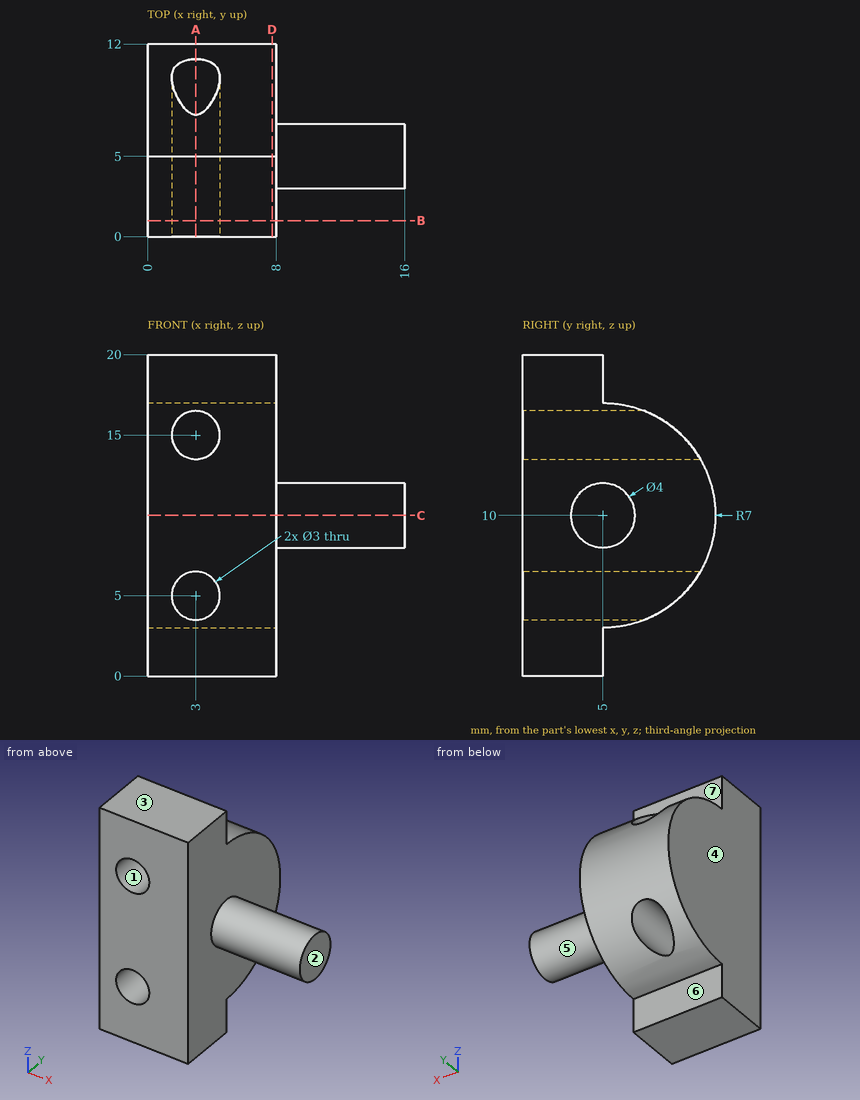
Study the drawing (mm; zero at the part's minimum x, y, z) and answer. A direction names the side the tool comes from. Coordinates: 2 decimals unless noted, no trailing zeros. Loops run counter-clockwise (first coordinate to the right, second up) from the corner with the lowest first, then second, coordinate; pieces in that order, holes last. Notation, with made-up numbers: (-38.75, -40) -> (-20.75, -40) arc R28 cw to (-20.75, -8) -> close; hole circle Ø2 at (1, 11.5). An arc over 180 degrees is marked (long way). Answer as CSV lines item,"result".
1) The part is cut by section D-D (x = 7.75). Give the vertices of the cut face in (y, z).
A:
outline,"(0, 0) -> (5, 0) -> (5, 3) arc R7 ccw to (5, 17) -> (5, 20) -> (0, 20) -> close"
2) For the marked faces 4, 5, 6 and 7, determine the directions among +Z, -Z, +X, -X, +Y, -Y from which every point of the face is accessible in a straight line to the end or side of a thin tool.
A:
face 4,"+Z, -Z, -X, +Y, -Y"
face 5,"+X"
face 6,"-Z, +X, -X, +Y"
face 7,"+Z, +X, -X, +Y"
3) Flat-ended cylindrical pins translate along their axes: pin 1 (3.5 mm diameter, centred on x = 5, z = 19, fed in from +Y); pin 2 (1 mm diameter, centred on x = 12.5, z = 12, fed in from -Y); pin 3 (1.5 mm diameter, centred on x = 12, y = 5.5, fed in from +Z); pin 4 (1.8 mm diameter, centred on x = 3, z = 5, fed in from +Y). Find the tip coordinate at first contact, or state that the pin passes through.
A:
pin 1,"stops at y = 5"
pin 2,"stops at y = 3.68"
pin 3,"stops at z = 12"
pin 4,"passes through"
4) The part is cut by section C-C (z = 10). Give the vertices of the cut face in (x, y), and give its area (3 significant figures).
A:
outline,"(0, 0) -> (8, 0) -> (8, 3) -> (16, 3) -> (16, 7) -> (8, 7) -> (8, 12) -> (0, 12) -> close"
area,"128 mm²"
5) The part is cut by section B-B (y = 1). Give the vertices of the cut face in (x, z), and give its area (3 significant figures).
A:
outline,"(0, 0) -> (8, 0) -> (8, 20) -> (0, 20) -> close; hole circle Ø3 at (3, 5); hole circle Ø3 at (3, 15)"
area,"146 mm²"
6) Straight lines are drawn through the part: probe 1 along X at (y, z) = (8.25, 15); probe 2 along Y at (x, z) = (3.75, 19); probe 3 along Z at (x, y) = (1.75, 2.5). For each, find the intervals that lie inside material, in ascending order.
A:
probe 1,"x = 0 to 1.5, 4.5 to 8"
probe 2,"y = 0 to 5"
probe 3,"z = 0 to 4.17, 5.83 to 14.17, 15.83 to 20"
7) The part is cut by section A-A (x = 3). Give the vertices of the cut face in (y, z), and give its area (3 significant figures).
A:
outline,"(0, 0) -> (5, 0) -> (5, 3) arc R7 ccw to (7.6, 3.5) -> (0, 3.5) -> close; (0, 6.5) -> (11.06, 6.5) arc R7 ccw to (11.06, 13.5) -> (0, 13.5) -> close; (0, 16.5) -> (7.6, 16.5) arc R7 ccw to (5, 17) -> (5, 20) -> (0, 20) -> close"
area,"119 mm²"
8) For a pull along Z with two mould halves and no side action, classify the marked faces 1, 2 and 3 as released by +Z, released by -Z, zero draft, split by the parting line, or undercut.
A:
face 1,"undercut"
face 2,"zero draft"
face 3,"released by +Z"
